Answer from the drawing. Dimensions are ordinates in mm from the lowest x, y and z of the part. A direction names the side the tool comes from. Round coordinates to 2 decimals unless told otherwise and drop trailing zeros. Write each loop counter-clockwise with the first axis right and the second up, starting at its lowest first coordinate (ties: lowest second). Pieces come first, ordered by that corner, then holes. Notation, with made-up numbers: (-17.5, -6.5) - (30.5, -6.5) arc R22 cw to (30.5, 5.5) - close; hole circle Ø11 at (86, 8). An arc over 180 degrees is marked (long way). One line per item, written item: value. Start each with the question number.
(1) The mould has two halves that part along X. Classify the marked faces 1, 2 and 3: +X half, -X half, draft (parallel to the pull), parting line (faces both ways), or undercut.
(2) Find the intervals of material crossed by L1, parallel to Y at x = 28, z = 1.9; L2, parallel to Y at x = 28, z = 3.75; L3, parallel to X at y = 25, z = 2.2, in increasing order.
(3) A cutting plane is placed at C-C, the plane z = 4.3. Determine the outline of the cut face in (x, y).
(4) For the marked faces 4 and 5, determine the directions among +Z, -Z, +X, -X, +Y, -Y from which every point of the face is accessible in a straight line to the end or side of a thin tool.
(5) A cutting plane is placed at A-A, the plane x = 28. Determine the outline of the cut face in (y, z), plus the area to 4 significant figures.
(6) Flat-ended cylindrical pins translate along their axes: pin 1 Ø5 at (x, y) = (25, 13) entering from -Z; pin 2 Ø1 at (y, z) = (40.5, 5.5) entering from -X; pin 3 Ø2 at (y, z) = (25.5, 1) entering from +X. Find the tip coordinate at first contact, or state that the pin passes through.
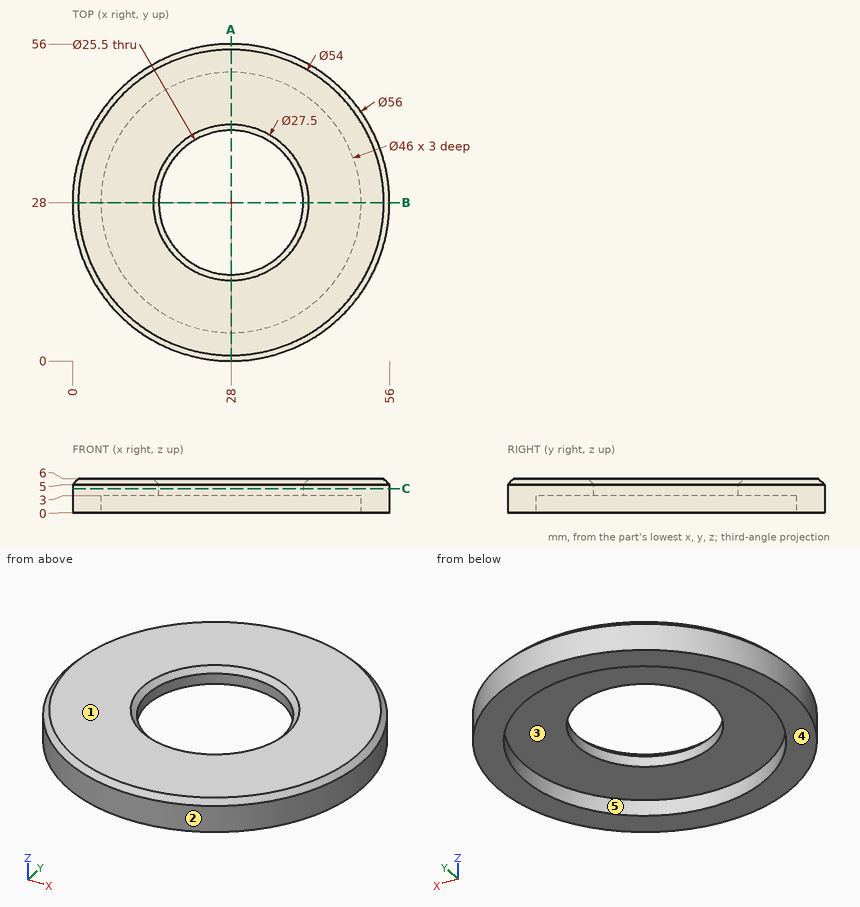
Here are the results:
1. face 1: draft
1. face 2: parting line
1. face 3: undercut
2. L1: 0 to 5, 51 to 56
2. L2: 0 to 15.25, 40.75 to 56
2. L3: 0.16 to 5.2, 50.8 to 55.84
3. outline: circle Ø56 at (28, 28); hole circle Ø25.5 at (28, 28)
4. face 4: -Z, +X, -X, +Y, -Y
4. face 5: -Z
5. outline: (0, 0) - (5, 0) - (5, 3) - (15.25, 3) - (15.25, 5) - (14.25, 6) - (1, 6) - (0, 5) - close; (40.75, 3) - (51, 3) - (51, 0) - (56, 0) - (56, 5) - (55, 6) - (41.75, 6) - (40.75, 5) - close
5. area: 119.5 mm²
6. pin 1: z = 3
6. pin 2: x = 2.89
6. pin 3: x = 55.96
